from build123d import *

# Parameters (mm, degrees)
BINDER_W                = 80
BINDER_H                = 50
PAD_DEPTH               = 3
BINDER001_W             = 12
BINDER001_H             = 3
PAD001_DEPTH            = 3
BINDER001_MIRRORED_2_W  = 12
BINDER001_MIRRORED_2_H  = 3
PAD001_MIRRORED_2_DEPTH = 3
LINEARPATTERN_COUNT     = 3
LINEARPATTERN_PITCH     = 22


with BuildPart() as part:
    # Binder → Pad (new body)
    with BuildSketch(Plane(origin=(47, 0, 0), x_dir=(0, -1, 0), z_dir=(1, 0, 0))):
        Rectangle(BINDER_W, BINDER_H)
    extrude(amount=PAD_DEPTH)

    # Binder001 → Pad001 (join)
    with BuildSketch(Plane(origin=(48.5, -22, 25), x_dir=(0, 1, 0), z_dir=(0, 0, 1))):
        Rectangle(BINDER001_W, BINDER001_H)
    pad001 = extrude(amount=PAD001_DEPTH)

    # Binder001 Mirrored 2 → Pad001 Mirrored 2 (add)
    with BuildSketch(Plane(origin=(48.5, -22, -25), x_dir=(0, 1, 0), z_dir=(0, 0, 1))):
        Rectangle(BINDER001_MIRRORED_2_W, BINDER001_MIRRORED_2_H)
    pad001_mirrored_2 = extrude(amount=-PAD001_MIRRORED_2_DEPTH)

    # LinearPattern: Pad001, Pad001 Mirrored 2 ×3
    with Locations(*[(0, i * LINEARPATTERN_PITCH, 0) for i in range(1, LINEARPATTERN_COUNT)]):
        add(pad001)
        add(pad001_mirrored_2)


solid = part.part
Part model, mm, in its own coordinate system. A direction names the side the tool comes from. Coordinates: 2 decimals unless noted, no trailing zeros. Write each loop counter-clockwise with the first axis right and the second up, starting at its lowest first coordinate (ties: lowest second). Pieces come first, ordered by that corner, then holes. Notation, with made-up numbers: M 20,-23.5 L 76,-23.5 A38 ccw 76,15.5 Z; hole C -12.75,-3.75 d5. An arc over 180 degrees is marked long. Return JSON: item names as keys, results as strings.
1. Saw through at B-B, the plane y = 29. Write the cut outline in (x, z), then the cut area to 3 significant figures.
Determined:
{"outline": "M 47,-25 L 50,-25 L 50,25 L 47,25 Z", "area": "150 mm²"}
2. Flat gauge pins, fed straight in: pin 1 Ø1.5 at (x, z) = (48, -27) entering from +Y; pin 2 Ø0.9 at (x, y) = (48, -12) entering from -Z; pin 3 Ø0.9 at (x, z) = (48, 26) entering from -Y. Where does each tip first touch, or does it go through?
Determined:
{"pin 1": "y = 28", "pin 2": "z = -25", "pin 3": "y = -28"}
3. Pull direction Y, two halves, no side cores. Call faces 1 (the face through (49, -28, -26)), 2 (the face through (49, 28, 26)), 3 (the face through (48, 0, 28)), 4 (the face through (49, 16, -26)): pulls with the +Y half, pulls with the -Y half, needs draft (parallel to the pull), parting line crosses it, or undercut.
Determined:
{"face 1": "pulls with the -Y half", "face 2": "pulls with the +Y half", "face 3": "needs draft", "face 4": "undercut"}
4. 3-axis set-ups, long thin cutter, end or side, ignore diameter. For faces 5 (the face through (49, 6, -26)), 6 (the face through (48, -34, 25)), 7 (the face through (48, -11, 25)): which of +Z, -Z, +X, -X, +Y, -Y reach the whole face in a straight line?
Determined:
{"face 5": "-Z, +X, -X", "face 6": "+Z, +X, -X, -Y", "face 7": "+Z, +X, -X"}
5. Probe L1, parallel to Z at x = 49.35, y = 28.5. List the from-to ranges inside material, lowest first.
Determined:
{"L1": "-25 to 25"}
6. Saw through at A-A, the plane x = 48.75. Write the cut outline in (y, z), then the cut area to 3 significant figures.
Determined:
{"outline": "M -40,-25 L -28,-25 L -28,-28 L -16,-28 L -16,-25 L -6,-25 L -6,-28 L 6,-28 L 6,-25 L 16,-25 L 16,-28 L 28,-28 L 28,-25 L 40,-25 L 40,25 L 28,25 L 28,28 L 16,28 L 16,25 L 6,25 L 6,28 L -6,28 L -6,25 L -16,25 L -16,28 L -28,28 L -28,25 L -40,25 Z", "area": "4,220 mm²"}
